```python
from build123d import *

# Parameters (mm, degrees)
PAD_DEPTH   = 12
FILLET_R    = 2
FILLET001_R = 2


with BuildPart() as part:
    # Sketch → Pad (new body)
    with BuildSketch(Plane.XZ):
        with BuildLine():
            Line((-35.492344, -2.005014), (-35.492339, 12.494989))
            ThreePointArc((-25.492339, 12.494987), (-30.492338, 17.494987), (-35.492339, 12.494989))
            Line((-25.492339, 12.494987), (-25.492339, -27.505013))
            ThreePointArc((-25.492339, -27.505013), (-19.294701, -34.891071), (-10.944645, -30.070164))
            Line((-10.944645, -30.070164), (0, 0))
            Line((0, 0), (-2.349232, 0.85505))
            Line((-2.349232, 0.85505), (-13.293876, -29.215114))
            ThreePointArc((-22.992339, -27.505013), (-18.86058, -32.429052), (-13.293876, -29.215114))
            Line((-22.992339, -27.505013), (-22.992339, 12.494987))
            ThreePointArc((-22.992339, 12.494987), (-30.492338, 19.994987), (-37.992339, 12.49499))
            Line((-37.992339, 12.49499), (-37.992344, -2.005013))
            ThreePointArc((-37.992344, -2.005013), (-37.628359, -3.672167), (-36.602644, -5.035911))
            Line((-36.602644, -5.035911), (-36.223782, -5.362198))
            Line((-36.223782, -5.362198), (-34.592345, -3.467888))
            Line((-34.592345, -3.467888), (-34.971207, -3.1416))
            ThreePointArc((-35.492344, -2.005014), (-35.35585, -2.630196), (-34.971207, -3.1416))
        make_face()
    extrude(amount=PAD_DEPTH)

    # Fillet
    fillet_edges = [part.edges().sort_by_distance(p)[0] for p in [
        (-1.174616, -12, 0.427525),
    ]]
    fillet(fillet_edges, radius=FILLET_R)

    # Fillet001
    fillet001_edges = [part.edges().sort_by_distance(p)[0] for p in [
        (-1.174616, 0, 0.427525),
    ]]
    fillet(fillet001_edges, radius=FILLET001_R)


solid = part.part
```
CAD build for the part. Positions are in the model's coordinates, mm. A direction names the side the tool comes from. Round coordinates to 2 decimals unless told otherwise and drop trailing zeros. Order: outer loops, then holes, each group sorted by start corner. A loop starts at its lowest first (then second) coordinate and runs counter-clockwise, first axis right, second up. Notation, with made-up numbers: (21, 12.5) - (61, 12.5) arc R27 cw to (61, 48.5) - close; hole circle Ø10 at (-0.75, 18). An arc over 180 degrees is marked (long way). Answer as CSV lines item,"result". Start each with the question number.
1. Drill centre lines: L1, parallel to X at y = -2, z = 12.5; L2, parallel to X at y = -8.5, z = -3.5; L3, parallel to X at y = -4, z = -3. Where is each one in solid material? Low to high. Write a range as [from, to].
2. Saw through at C-C, the plane z = -13. Write the cut outline in (x, y).
3. Saw through at A-A, the plane z = 5.5. Write the cut outline in (x, y), and give its area (3 significant figures).
4. Saw through at B-B, the plane y = -6.75. Write the cut outline in (x, z) (3 decimals), and give its area (3 significant figures).
5. Pull direction Z, two halves, no side cores. Call faces 1 (the face through (-1.4, -11.4, -0.1)), 2 (the face through (-35.42, -5.92, -4.43)), 3 (the face through (-35.36, -5.92, -2.62)): +Z half, -Z half, draft (parallel to the pull), parting line (faces both ways), or undercut.
6. Saw through at D-D, the plane x = -29. Write the cut outline in (y, z), and give its area (3 significant figures).
7. Pin check, flat tips, straight feed: pin 1 (5 mm diameter, centred on y = -7, z = -24.5, fed in from -X); pin 2 (2 mm diameter, centred on y = -10, z = -29, fed in from +X); pin 3 (6 mm diameter, centred on y = -3.5, z = 4, fed in from +X). Stop position of each tip, or through.
8. Tool access for faces 4 (the face through (-35.492, -6, 5)), 5 (the face through (-25.492, -6, -7)), 6 (the face through (-22.992, -6, -8)), 7 (the face through (-37.64, -5.92, -3.65)), 8 (the face through (-24, -12, -5)): list every direction of +Z, -Z, +X, -X, +Y, -Y with a clear straight run to the whole face (end or side of a thin tool).
Model answer:
1,L1,"x = [-37.99, -35.49], [-25.49, -22.99]"
1,L2,"x = [-37.7, -34.62], [-25.49, -22.99], [-3.93, -1.27]"
1,L3,"x = [-37.87, -35.11], [-25.49, -22.99], [-3.75, -1.09]"
2,outline,"(-25.49, -12) - (-22.99, -12) - (-22.99, 0) - (-25.49, 0) - close; (-7.39, -12) - (-4.73, -12) - (-4.73, 0) - (-7.39, 0) - close"
3,outline,"(-37.99, -12) - (-35.49, -12) - (-35.49, 0) - (-37.99, 0) - close; (-25.49, -12) - (-22.99, -12) - (-22.99, 0) - (-25.49, 0) - close"
3,area,"60.0 mm²"
4,outline,"(-37.992, -2.005) arc R4 ccw to (-36.603, -5.036) - (-36.224, -5.362) - (-34.592, -3.468) - (-34.971, -3.142) arc R1.5 cw to (-35.492, -2.005) - (-35.492, 12.495) arc R5 cw to (-25.492, 12.495) - (-25.492, -27.505) arc R7.5 ccw to (-10.945, -30.07) - (0, 0) - (-2.349, 0.855) - (-13.294, -29.215) arc R5 cw to (-22.992, -27.505) - (-22.992, 12.495) arc R7.5 ccw to (-37.992, 12.495) - close"
4,area,"316 mm²"
5,face 1,"+Z half"
5,face 2,"-Z half"
5,face 3,"undercut"
6,outline,"(-12, 17.27) - (0, 17.27) - (0, 19.85) - (-12, 19.85) - close"
6,area,"30.9 mm²"
7,pin 1,"stops at x = -25.49"
7,pin 2,"stops at x = -10.19"
7,pin 3,"stops at x = -22.99"
8,face 4,"+Y, -Y"
8,face 5,"-Z, +Y, -Y"
8,face 6,"+Z, +Y, -Y"
8,face 7,"-Z, -X, +Y, -Y"
8,face 8,"+Z, -Z, +X, -X, -Y"
